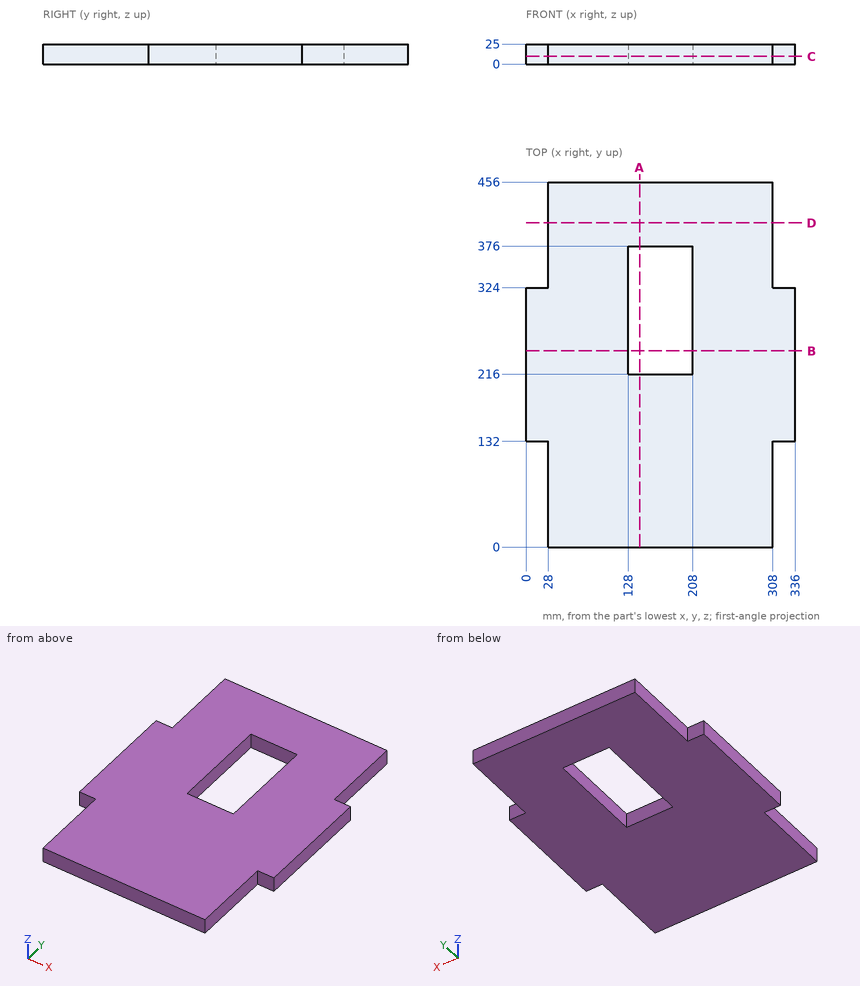
Design review of the part shown in the three views and the two pictorial views. Dimensions are in mm from the part's minimum x, y and z. Give positions to 0.01 mm unless a question says otherwise; leave off trailing zeros. Write each loop counter-clockwise with the first axis right and the second up, starting at its lowest first coordinate (ties: lowest second). Pieces come first, ordered by that corner, then holes.
(1) Add section C-C (z = 9.5). Give the boundary of the cut face in (x, y), and give its area (3 significant figures).
Checked values:
outline: (0, 132) - (28, 132) - (28, 0) - (308, 0) - (308, 132) - (336, 132) - (336, 324) - (308, 324) - (308, 456) - (28, 456) - (28, 324) - (0, 324) - close; hole (128, 216) - (208, 216) - (208, 376) - (128, 376) - close
area: 126,000 mm2
(2) Wall thickness on line 1 along X through (y, z) = (226.5, 4.5); line 2 along Y through (x, z) = (144, 4.5); line 3 along X through (y, z) = (374.5, 16.25): over which ranges is each line inside the solid? List them lowest first.
Checked values:
line 1: x = 0 to 128, 208 to 336
line 2: y = 0 to 216, 376 to 456
line 3: x = 28 to 128, 208 to 308
(3) Add section B-B (y = 245). Give the boundary of the cut face in (x, z), and give its area (3 significant figures).
Checked values:
outline: (0, 0) - (128, 0) - (128, 25) - (0, 25) - close; (208, 0) - (336, 0) - (336, 25) - (208, 25) - close
area: 6,400 mm2
(4) Add section D-D (y = 405). Give the boundary of the cut face in (x, z), and give its area (3 significant figures).
Checked values:
outline: (28, 0) - (308, 0) - (308, 25) - (28, 25) - close
area: 7,000 mm2
(5) Clearance check with flat-ended pins moving along their axes: pin 1 Ø1.5 at (y, z) = (292, 12) entering from -X; pin 2 Ø3 at (y, z) = (96, 2.5) entering from -X; pin 3 Ø7.5 at (x, z) = (19.5, 16) entering from -Y; pin 4 Ø7.5 at (y, z) = (368.5, 14) entering from +X. State where each tip first meets the part, or that it passes through.
Checked values:
pin 1: stops at x = 0
pin 2: stops at x = 28
pin 3: stops at y = 132
pin 4: stops at x = 308
(6) Add section A-A (x = 142). Give the boundary of the cut face in (y, z), and give its area (3 significant figures).
Checked values:
outline: (0, 0) - (216, 0) - (216, 25) - (0, 25) - close; (376, 0) - (456, 0) - (456, 25) - (376, 25) - close
area: 7,400 mm2
